Autodesk Inventor part; units mm, degrees
ref_plane "YZ Plane" through (0, 0, 0) normal (1, 0, 0) x (0, 1, 0)
ref_plane "XZ Plane" through (0, 0, 0) normal (0, 1, 0) x (-1, 0, 0)
ref_plane "XY Plane" through (0, 0, 0) normal (0, 0, 1) x (1, 0, 0)
sketch "Sketch1" plane through (0, 0, 0) normal (0, 1, 0) x (-1, 0, 0)
  line L0 (-26.5, -50) -> (26.5, -50)
  line L1 (26.5, -50) -> (26.5, 50)
  line L2 (26.5, 50) -> (-26.5, 50)
  line L3 (-26.5, 50) -> (-26.5, -50)
  line L4 (-26.5, -50) -> (26.5, 50) construction
  line L5 (26.5, -50) -> (-26.5, 50) construction
  point P0 (0, 0)
  dimension "d0" = 53
  dimension "d1" = 100
extrude "Extrusion1" add sketch "Sketch1" along normal blind 1.2
sketch "Sketch2" plane through (26.5, 0, 50) normal (1, 0, 0) x (0, 0, -1)
  line L0 (100, 0) -> (0, 0)
  line L1 (0, 0) -> (100, 0)
  line L2 (100, 0) -> (100, 9)
  line L3 (100, 9) -> (0, 9)
  line L4 (0, 9) -> (0, 0)
  point P0 (50, 0)
  dimension "d4" = 9
extrude "Extrusion2" add sketch "Sketch2" along normal blind 2
sketch "Sketch3" plane through (26.5, 1.2, 50) normal (0, 0, 1) x (1, 0, 0)
  line L0 (-53, -1.2) -> (2, -1.2)
  line L1 (2, 7.8) -> (2, -1.2)
  line L2 (0, 7.8) -> (2, 7.8)
  line L3 (0, 7.8) -> (0, 0)
  line L4 (-53, 0) -> (0, 0)
  line L5 (-53, -1.2) -> (-53, 0)
  line L6 (0, 7.8) -> (2, 7.8)
  line L7 (-53, 0) -> (0, 7.8)
  point P0 (-26.5, -1.2)
extrude "Extrusion3" add sketch "Sketch3" along normal blind 1.5
mirror "Mirror1" about plane through (0, 0, 0) normal (0, 0, 1) of "Extrusion3"
sketch "Sketch4" plane through (26.5, 0, 50) normal (-1, 0, 0) x (0, 0, 1)
  line L0 (0, 1.2) -> (-100, 1.2)
  line L1 (0, 9) -> (0, 1.2)
  line L2 (-100, 9) -> (0, 9)
  line L3 (-100, 1.2) -> (-100, 9)
  line L4 (-5, 5.1) -> (-95, 5.1)
  line L5 (-100, 1.2) -> (0, 1.2)
  point P0 (-50, 0)
  point P1 (0, 5.1)
  point P2 (-50, 5.1)
  point P3 (-50, 9)
  dimension "d9" = 90
hole "Hole1" at (26.5, 5.1, 45) at (26.5, 5.1, 0) at (26.5, 5.1, -45) direction (1, 0, 0) diameter 2.4 end through all
sketch "Sketch5" plane through (0, 1.2, 0) normal (0, 1, 0) x (1, 0, 0)
  circle A0 centre (-1.5, -25) radius 23
  line L0 (18.5, -5) -> (-21.5, -5)
  line L1 (-21.5, -5) -> (-21.5, -45)
  line L2 (-21.5, -45) -> (18.5, -45)
  line L3 (18.5, -45) -> (18.5, -5)
  line L4 (18.5, -5) -> (-21.5, -45) construction
  line L5 (-21.5, -5) -> (18.5, -45) construction
  line L6 (-26.5, 50) -> (-26.5, -50)
  point P0 (0, 0)
  dimension "d17" = 46
  dimension "d18" = 40
  dimension "d19" = 40
  dimension "d20" = 25
  dimension "d21" = 25
extrude "Extrusion4" cut sketch "Sketch5" against normal through all contours A0 L3 | L3 A0 L2 L1 L0 | L0 A0 | A0 L2 | L1 A0
hole "Hole2" at (-21.5, 1.2, 45) at (-21.5, 1.2, 5) at (18.5, 1.2, 5) at (18.5, 1.2, 45) direction (0, -1, 0) diameter 3.2 end through all
mirror "Mirror2" about plane through (0, 0, 0) normal (0, 0, 1) of "Hole2", "Extrusion4"
equation "\"d19\" = d18"
properties part number "Fan_Bracket"
Geometry check sheet. Reference: the model listing, model coordinates, mm. A direction names the side the tool comes from. Coordinates: 2 decimals unless noted, no trailing zeros. Write each loop counter-clockwise with the first axis right and the second up, starting at its lowest first coordinate (ties: lowest second). Pieces come first, ordered by that corner, then holes. Notation, with made-up numbers: M 76.5,-3 L 88.5,-3 A24 cw 88.5,35 Z; hole C 76.25,-2 d1. An arc over 180 degrees is marked long. One line per item, written item: value. Start each with the question number.
(1) Sectioned sample at B-B, the plane x = -1.5. Enter the section's corners in (y, z).
(2) Tool access check on faces 1 (the face through (-23.086, 0.592, 44.792)), 2 (the face through (26.5, 3, 1)). Record the directions out of +Z, -Z, +X, -X, +Y, -Y that give a thin tool (end or side, any length) a straight path to the whole face; none if there is none.
(3) Release check for a two-part mould opening along Z. For faces 3 (the face through (12, 3, -50)), 4 (the face through (7, 4, 51.5)), 5 (the face through (11, 3, 50)), 6 (the face through (28.5, 4, 1)) record: released by +Z, released by -Z, zero draft, split by the parting line, or undercut.
(4) Sectioned sample at A-A, the plane z = -25. Enter the section's corners in (x, y), and give its area (3 significant figures).
(5) Sectioned sample at D-D, the plane z = -45. Enter the section's corners in (x, y).
(6) Depth check by flat-ended pin: pin 1 (2.5 mm diameter, centred on y = 6, z = -24, fed in from -X). Enter the tip coordinate at first touch or a pass-through.
(7) Sectioned sample at C-C, the plane z = 5. Enter the section's corners in (x, y), and give its area (3 significant figures).
(8) Scan lines: line 1 along Z through (x, y) = (-1.5, 0.8); line 2 along Z through (x, y) = (-4, 1.5); line 3 along X through (y, z) = (0.8, 45). Record each from-to range of solid material in increasing order. Write a range as [from, to].
Filled sheet:
1. outline: M 0,-51.5 L 4.88,-51.5 L 4.88,-50 L 1.2,-50 L 1.2,-48 L 0,-48 Z; M 0,-2 L 1.2,-2 L 1.2,2 L 0,2 Z; M 0,48 L 1.2,48 L 1.2,50 L 4.88,50 L 4.88,51.5 L 0,51.5 Z
2. face 1: +Y, -Y
2. face 2: -X, +Y
3. face 3: undercut
3. face 4: released by +Z
3. face 5: undercut
3. face 6: zero draft
4. outline: M -26.5,0 L -24.5,0 L -24.5,1.2 L -26.5,1.2 Z; M 21.5,0 L 28.5,0 L 28.5,9 L 26.5,9 L 26.5,1.2 L 21.5,1.2 Z
4. area: 26.4 mm²
5. outline: M -26.5,0 L -23.1,0 L -23.1,1.2 L -26.5,1.2 Z; M -19.9,0 L -12.86,0 L -12.86,1.2 L -19.9,1.2 Z; M 9.86,0 L 16.9,0 L 16.9,1.2 L 9.86,1.2 Z; M 20.1,0 L 28.5,0 L 28.5,3.9 L 26.5,3.9 L 26.5,1.2 L 20.1,1.2 Z; M 26.5,6.3 L 28.5,6.3 L 28.5,9 L 26.5,9 Z
6. pin 1: x = 26.5
7. outline: M -26.5,0 L -23.1,0 L -23.1,1.2 L -26.5,1.2 Z; M -19.9,0 L -12.86,0 L -12.86,1.2 L -19.9,1.2 Z; M 9.86,0 L 16.9,0 L 16.9,1.2 L 9.86,1.2 Z; M 20.1,0 L 28.5,0 L 28.5,9 L 26.5,9 L 26.5,1.2 L 20.1,1.2 Z
7. area: 46.7 mm²
8. line 1: [-51.5, -48], [-2, 2], [48, 51.5]
8. line 2: [-51.5, -50], [50, 51.5]
8. line 3: [-26.5, -23.1], [-19.9, -12.86], [9.86, 16.9], [20.1, 28.5]
